from build123d import *

# Parameters (mm, degrees)
F0_R     = 1.5875
F0_R_2   = 3.175
F1_DEPTH = 13
F2_W     = 6.35
F2_H     = 19.05
F3_DEPTH = 37.5
F4_R     = 10
F5_R     = 5
F6_SIZE  = 1
F7_SIZE  = 3.175


with BuildPart() as f1:
    # F0 (on Right) → F1 (new body)
    with BuildSketch(Plane.YZ):
        Polygon((0, 31.75), (0, 0), (0, -31.75), (19.05, -31.75), (63.5, -12.7), (92.075, -12.7), (92.075, 0), (92.075, 12.7), (63.5, 12.7), (19.05, 31.75), align=None)
        with Locations((9.525, -15.875)):
            Circle(F0_R, mode=Mode.SUBTRACT)
        with Locations((41.275, 0)):
            Circle(F0_R_2, mode=Mode.SUBTRACT)
        with Locations((9.525, 15.875)):
            Circle(F0_R, mode=Mode.SUBTRACT)
        with Locations((82.55, 0)):
            Circle(F0_R, mode=Mode.SUBTRACT)
    extrude(amount=-F1_DEPTH)

    # F2 (on Top) → F3 (cut, symmetric)
    with BuildSketch(Plane.XY):
        with BuildLine():
            Line((0, 30.276477), (0, 52.273523))
            ThreePointArc((0, 52.273523), (-6.35, 41.275), (0, 30.276477))
        make_face()
        with Locations((-3.175, 82.55)):
            Rectangle(F2_W, F2_H)
    extrude(amount=F3_DEPTH, both=True, mode=Mode.SUBTRACT)

    # F4
    f4_edges = [f1.edges().sort_by_distance(p)[0] for p in [
        (-6.5, 19.05, 31.75),
        (-6.5, 63.5, 12.7),
        (-6.5, 63.5, -12.7),
        (-6.5, 19.05, -31.75),
    ]]
    fillet(f4_edges, radius=F4_R)

    # F5
    f5_edges = [f1.edges().sort_by_distance(p)[0] for p in [
        (-13, 92.075, 0),
        (0, 0, 0),
    ]]
    fillet(f5_edges, radius=F5_R)

    # F6
    f6_edges = [f1.edges().sort_by_distance(p)[0] for p in [
        (-13, 76.313789, 12.7),
        (0, 10.998711, 31.75),
        (0, 25.606547, 28.940051),
        (0, 56.943453, 15.509949),
        (0, 69.288789, -12.7),
        (0, 25.606547, -28.940051),
        (0, 56.943453, -15.509949),
        (-13, 76.313789, -12.7),
    ]]
    chamfer(f6_edges, length=F6_SIZE)

    # F7
    f7_edges = [f1.edges().sort_by_distance(p)[0] for p in [
        (-13, 38.1, 0),
    ]]
    chamfer(f7_edges, length=F7_SIZE)


solid = f1.part
Read the model definition and answer for the solid it produces. Units are mm, in the model's axes. A direction names the side the tool comes from. Give positions to 0.01 mm unless a question says otherwise; leave off trailing zeros. Loops run counter-clockwise (first coordinate to the right, second up) from the corner with the lowest first, then second, coordinate; pieces in that order, holes last. Notation, with made-up numbers: (-24.75, -32) - (-10.75, -32) arc R8 cw to (-10.75, -23) - close; hole circle Ø3 at (41.25, -10.75). An arc over 180 degrees is marked (long way). Answer as CSV lines item,"result". Start each with the question number.
1) Determine the mould class of faces 1 (the face through (-12.49, 63.41, -12.43)), 2 (the face through (-7.86, 40.59, -3.1)), 3 (the face through (-6.409, 8.265, -16.841)), 4 (the face through (0, 63, 0)) for opening direction Y: released by +Y, released by -Y, zero draft, split by the parting line, or undercut.
2) Each of these flat-tipped pins is pushed along its axis until it touches: pin 1 Ø4 at (y, z) = (82.55, 0) entering from +X; pin 2 Ø6 at (y, z) = (73.5, -5.5) entering from +X; pin 3 Ø3 at (x, y) = (-5, 31.5) entering from +Z; pin 4 Ø1.5 at (x, z) = (-2, -20) entering from +Y. Where does it stop, or does it pass through?
3) Find section B-B (z = 0). State how many separate pieces and enclosed holes the cut face has, then the cut area to 3 significant figures.
4) Find section C-C (y = 68). Write down the section's boundary in (x, z), then the cut area to 3 significant figures.
5) Which of the six approach directions +Z, -Z, +X, -X, +Y, -Y give full straight-line access (tool end or side, diameter ignored) to faces 5 (the face through (-3, 73.025, 0)), 6 (the face through (-8, 75, -12.7)), 7 (the face through (-6, 9, 31.75))?
6) Straight lines are drawn through the part: L1, parallel to Z at x = -11.5, y = 10.5; L2, parallel to Z at x = -7.5, y = 75; L3, parallel to Z at x = -3.5, y = 8.5. For each, find the intervals that lie inside material, in ascending order. Write a range as from..to.
7) Find section D-D (z = 8). Write down the section's boundary in (x, y) (3 decimals).
8) Find section A-A (y = 82.55). Write down the section's boundary in (x, z).
Findings below:
1,face 1,"released by +Y"
1,face 2,"undercut"
1,face 3,"undercut"
1,face 4,"zero draft"
2,pin 1,"x = -6.35"
2,pin 2,"x = 0"
2,pin 3,"z = 27.06"
2,pin 4,"y = 32.42"
3,separate pieces,"3"
3,enclosed holes,"0"
3,area,"892 mm^2"
4,outline,"(-13, -11.7) - (-12, -12.7) - (-1, -12.7) - (0, -11.7) - (0, 11.7) - (-1, 12.7) - (-12, 12.7) - (-13, 11.7) - close"
4,area,"328 mm^2"
5,face 5,"+Z, -Z, +X, +Y"
5,face 6,"-Z, +X, -X, +Y"
5,face 7,"+Z, +X, -X, +Y, -Y"
6,L1,"-31.75..-17.13, -14.62..14.62, 17.13..31.75"
6,L2,"-12.7..12.7"
6,L3,"-31.75..-17.09, -14.66..14.66, 17.09..31.75"
7,outline,"(-13, 0) - (-5, 0) arc R5 ccw to (0, 5) - (0, 30.276) arc R12.7 cw to (0, 52.274) - (0, 73.025) - (-6.35, 73.025) - (-6.35, 92.075) - (-8, 92.075) arc R5 ccw to (-13, 87.075) - close"
8,outline,"(-13, -11.7) - (-12, -12.7) - (-6.35, -12.7) - (-6.35, -1.59) - (-13, -1.59) - close; (-13, 1.59) - (-6.35, 1.59) - (-6.35, 12.7) - (-12, 12.7) - (-13, 11.7) - close"
